Can you work these out from the model? Positions are in its coordinate system, mm. Face numbers are marked on the shaded views. A direction names the side the tool comes from. Round coordinates to 2 decimals unless told otherwise and drop trailing zeros. Loops run counter-clockwise (first coordinate to the right, second up) from the corner with the lowest first, then second, coordinate; pieces in that order, holes last. Notation, with made-up numbers: M -33.5,2.5 L -9.5,2.5 A32 ccw -9.5,37.5 Z; hole C 21,35 d9. An arc over 180 degrees is marked long. Answer as CSV lines item,"result".
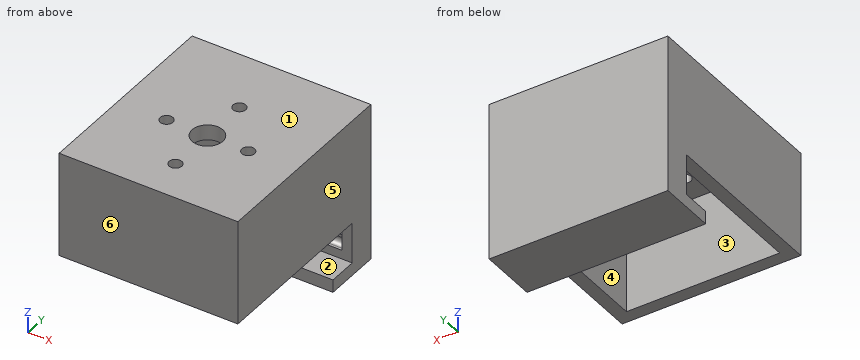
from build123d import *

# Parameters (mm, degrees)
SKETCH1_R           = 1.25
SKETCH1_R_2         = 3
BOSS_EXTRUDE1_DEPTH = 3
SKETCH2_W           = 35
SKETCH2_H           = 39.5
SKETCH2_W_2         = 30
SKETCH2_H_2         = 30
BOSS_EXTRUDE2_DEPTH = 20.55
BOSS_EXTRUDE3_START = -3
SKETCH2_2_W         = 30
SKETCH2_2_H         = 30
BOSS_EXTRUDE3_DEPTH = 3
SKETCH3_W           = 35
SKETCH3_H           = 11.242333622
BOSS_EXTRUDE4_DEPTH = 10.5
CUT_EXTRUDE1_REACH  = 51.958
SKETCH4_W           = 8
SKETCH4_H           = 5.717333622
CUT_EXTRUDE2_START  = -33
CUT_EXTRUDE2_DEPTH  = 31


with BuildPart() as part:
    # Sketch1 → Boss-Extrude1 (new body)
    with BuildSketch(Plane.XY):
        with BuildLine():
            Line((-10.880679664, -4.940982702), (-10.677312396, -4.737615434))
            ThreePointArc((-10.677312396, -4.737615434), (-4.737615434, -4.737615434), (-4.737615434, -10.677312396))
            Line((-4.737615434, -10.677312396), (-4.940982702, -10.880679664))
            ThreePointArc((-4.940982702, -10.880679664), (0, -11.95), (4.940982702, -10.880679664))
            Line((4.940982702, -10.880679664), (4.737615434, -10.677312396))
            ThreePointArc((4.737615434, -10.677312396), (4.737615434, -4.737615434), (10.677312396, -4.737615434))
            Line((10.677312396, -4.737615434), (10.880679664, -4.940982702))
            ThreePointArc((10.880679664, -4.940982702), (11.95, 0), (10.880679664, 4.940982702))
            Line((10.880679664, 4.940982702), (10.677312396, 4.737615434))
            ThreePointArc((10.677312396, 4.737615434), (4.737615434, 4.737615434), (4.737615434, 10.677312396))
            Line((4.737615434, 10.677312396), (4.940982702, 10.880679664))
            ThreePointArc((4.940982702, 10.880679664), (0, 11.95), (-4.940982702, 10.880679664))
            Line((-4.940982702, 10.880679664), (-4.737615434, 10.677312396))
            ThreePointArc((-4.737615434, 10.677312396), (-4.737615434, 4.737615434), (-10.677312396, 4.737615434))
            Line((-10.677312396, 4.737615434), (-10.880679664, 4.940982702))
            ThreePointArc((-10.880679664, 4.940982702), (-11.95, 0), (-10.880679664, -4.940982702))
        make_face()
        with Locations((8, 0)):
            Circle(SKETCH1_R, mode=Mode.SUBTRACT)
        with Locations((0, 9.5)):
            Circle(SKETCH1_R, mode=Mode.SUBTRACT)
        with Locations((0, -9.5)):
            Circle(SKETCH1_R, mode=Mode.SUBTRACT)
        with Locations((-8, 0)):
            Circle(SKETCH1_R, mode=Mode.SUBTRACT)
        Circle(SKETCH1_R_2, mode=Mode.SUBTRACT)
    extrude(amount=BOSS_EXTRUDE1_DEPTH)



with BuildPart() as body_2:
    # Sketch2 → Boss-Extrude2 (new body)
    with BuildSketch(Plane.XY.offset(3)):
        with Locations((0, 2.25)):
            Rectangle(SKETCH2_W, SKETCH2_H)
        Rectangle(SKETCH2_W_2, SKETCH2_H_2, mode=Mode.SUBTRACT)
    extrude(amount=-BOSS_EXTRUDE2_DEPTH)


with BuildPart() as part_1:
    add(part.part)

    add(body_2.part)  # Boss-Extrude3 merges body 2
    # Sketch2<2> → Boss-Extrude3 (add)
    with BuildSketch(Plane.XY.offset(3).offset(BOSS_EXTRUDE3_START)):
        Rectangle(SKETCH2_2_W, SKETCH2_2_H)
        with BuildLine():
            ThreePointArc((-10.880679664, 4.940982702), (-11.95, 0), (-10.880679664, -4.940982702))
            Line((-10.880679664, -4.940982702), (-10.677312396, -4.737615434))
            ThreePointArc((-10.677312396, -4.737615434), (-4.737615434, -4.737615434), (-4.737615434, -10.677312396))
            Line((-4.737615434, -10.677312396), (-4.940982702, -10.880679664))
            ThreePointArc((-4.940982702, -10.880679664), (0, -11.95), (4.940982702, -10.880679664))
            Line((4.940982702, -10.880679664), (4.737615434, -10.677312396))
            ThreePointArc((4.737615434, -10.677312396), (4.737615434, -4.737615434), (10.677312396, -4.737615434))
            Line((10.677312396, -4.737615434), (10.880679664, -4.940982702))
            ThreePointArc((10.880679664, -4.940982702), (11.95, 0), (10.880679664, 4.940982702))
            Line((10.880679664, 4.940982702), (10.677312396, 4.737615434))
            ThreePointArc((10.677312396, 4.737615434), (4.737615434, 4.737615434), (4.737615434, 10.677312396))
            Line((4.737615434, 10.677312396), (4.940982702, 10.880679664))
            ThreePointArc((4.940982702, 10.880679664), (0, 11.95), (-4.940982702, 10.880679664))
            Line((-4.940982702, 10.880679664), (-4.737615434, 10.677312396))
            ThreePointArc((-4.737615434, 10.677312396), (-4.737615434, 4.737615434), (-10.677312396, 4.737615434))
            Line((-10.677312396, 4.737615434), (-10.880679664, 4.940982702))
        make_face(mode=Mode.SUBTRACT)
    extrude(amount=BOSS_EXTRUDE3_DEPTH)

    # Sketch3 → Boss-Extrude4 (add)
    with BuildSketch(Plane(origin=(0, 0, -17.55), x_dir=(-1, 0, 0), z_dir=(0, 0, -1))):
        with Locations((0, 16.378833189)):
            Rectangle(SKETCH3_W, SKETCH3_H)
    extrude(amount=BOSS_EXTRUDE4_DEPTH)

    # Sketch4 → Cut-Extrude1 (cut, up to next)
    with BuildSketch(Plane(origin=(17.5, 0, 0), x_dir=(0, 0, -1), z_dir=(1, 0, 0)), mode=Mode.PRIVATE) as cut_extrude1_sk1:
        with Locations((21.55, 13.616333189)):
            Rectangle(SKETCH4_W, SKETCH4_H)
    cut_extrude1_tool1 = extrude(cut_extrude1_sk1.sketch, amount=-CUT_EXTRUDE1_REACH, mode=Mode.PRIVATE) & part_1.part
    add(cut_extrude1_tool1.solids().sort_by_distance((17.5, 13.616333, -21.55))[0], mode=Mode.SUBTRACT)

    # Sketch4<3> → Cut-Extrude2 (cut)
    with BuildSketch(Plane(origin=(17.5, 0, 0), x_dir=(0, 0, -1), z_dir=(1, 0, 0)).offset(CUT_EXTRUDE2_START)):
        with BuildLine():
            Line((21.55, 17.175), (21.55, 16.475))
            Line((21.55, 16.475), (23.8, 16.475))
            Line((23.8, 16.475), (23.8, 16.975))
            ThreePointArc((23.8, 16.975), (22.900508962, 17.969936153), (21.820204103, 17.175))
            Line((21.820204103, 17.175), (21.55, 17.175))
        make_face()
        with BuildLine():
            Line((19.3, 16.975), (19.3, 16.475))
            Line((19.3, 16.475), (21.55, 16.475))
            Line((21.55, 16.475), (21.55, 17.175))
            Line((21.55, 17.175), (21.279795897, 17.175))
            ThreePointArc((21.279795897, 17.175), (20.199491038, 17.969936153), (19.3, 16.975))
        make_face()
    extrude(amount=CUT_EXTRUDE2_DEPTH, mode=Mode.SUBTRACT)


solid = part_1.part
Item 1: If we section it at B-B on x = 0: State how many separate pieces and enclosed holes the cut face has, then the cut area to 3 significant figures.
Output:
separate pieces,"4"
enclosed holes,"0"
area,"319 mm2"
Item 2: If we section it at C-C on x = 8: Write out the boundary of the cut face in (y, z) (3 decimals).
Output:
outline,"M -17.5,-17.55 L -15,-17.55 L -15,0 L -1.25,0 L -1.25,3 L -17.5,3 Z; M 1.25,0 L 15,0 L 15,-17.55 L 16.475,-17.55 L 16.475,-19.3 L 16.975,-19.3 A1 cw 17.175,-21.28 L 17.175,-21.82 A1 cw 16.975,-23.8 L 16.475,-23.8 L 16.475,-25.55 L 10.758,-25.55 L 10.758,-28.05 L 22,-28.05 L 22,3 L 1.25,3 Z"
Item 3: Will these pins go through, and if not, where does the flat tip stop? pin 1 (15 mm diameter, centred on x = -4, y = 1, fed in from -Z); pin 2 (0.8 mm diameter, centred on x = 2, z = -26.5, fed in from -Y); pin 3 (0.6 mm diameter, centred on x = 3, z = -21.5, fed in from -Y) (3 decimals).
Output:
pin 1,"stops at z = 0"
pin 2,"stops at y = 10.76"
pin 3,"stops at y = 17.175"
Item 4: On a 3-axis mill with a long thin cutter (end or side, diameter ignored), from which of +Z, -Z, +X, -X, +Y, -Y can I reach the whole of each face in a straight line? I mean the marked faces 1, 2 and 3. Say none if no direction works.
Output:
face 1,"+Z, +X, -X, +Y, -Y"
face 2,"+X, -X, -Y"
face 3,"-Z"
Item 5: If we section it at A-A on y = 0: Write out the boundary of the cut face in (x, z).
Output:
outline,"M -17.5,-17.55 L -15,-17.55 L -15,0 L -9.25,0 L -9.25,3 L -17.5,3 Z; M -6.75,0 L -3,0 L -3,3 L -6.75,3 Z; M 3,0 L 6.75,0 L 6.75,3 L 3,3 Z; M 9.25,0 L 15,0 L 15,-17.55 L 17.5,-17.55 L 17.5,3 L 9.25,3 Z"
Item 6: If I drill on line 1 along Y through (x, z) = (0, 1.1); line 2 along Y through (x, z) = (12, -2.5); line 3 along X through (y, z) = (11, -10), over which ranges is the centre line in solid material (lowest first)? Write a range as from..to.
Output:
line 1,"y = -17.5..-10.75, -8.25..-3, 3..8.25, 10.75..22"
line 2,"y = -17.5..-15, 15..22"
line 3,"x = -17.5..-15, 15..17.5"
Item 7: We'd pull the mould along X, two halves only. Please class the marked faces 4, 5 and 6: released by +X, released by -X, zero draft, split by the parting line, or undercut.
Output:
face 4,"undercut"
face 5,"released by +X"
face 6,"zero draft"
Item 8: If we section it at D-D on y = -9.5: Write out the boundary of the cut face in (x, z), then the cut area to 3 significant figures.
Output:
outline,"M -17.5,-17.55 L -15,-17.55 L -15,0 L -1.25,0 L -1.25,3 L -17.5,3 Z; M 1.25,0 L 15,0 L 15,-17.55 L 17.5,-17.55 L 17.5,3 L 1.25,3 Z"
area,"185 mm2"
